CAD build for the part. Positions are in the model's coordinates, mm. A direction names the side the tool comes from. Coordinates: 2 decimals unless noted, no trailing zeros. Order: outer loops, then holes, each group sorted by start corner. A loop starts at its lowest first (then second) coordinate and runs counter-clockwise, first axis right, second up. Notation, with made-up numbers: M -12.75,63 L 32.25,63 A24 ccw 32.25,85 Z; hole C -21,-8.5 d2. An arc over 180 degrees is marked long. Write item = value, one per line. Start each with the question number.
```python
from build123d import *

# Parameters (mm, degrees)
SKETCH1_R               = 1.5875
BOSS_EXTRUDE1_DEPTH     = 22.86
TOP_CUT_DEPTH           = 8.255
BOTTOM_CUT_DEPTH        = 8.255
SKETCH5_R               = 10.033
CUT_EXTRUDE1_DEPTH      = 14.986
SKETCH7_R               = 2.032
CUT_EXTRUDE2_DEPTH      = 49.946539324
CUT_EXTRUDE3_REACH      = 50.947
CUT_EXTRUDE3_END_RADIUS = 10.033
SKETCH8_W               = 3.175
SKETCH8_H               = 6.35


with BuildPart() as part:
    # Sketch1 → Boss-Extrude1 (new body)
    with BuildSketch(Plane(origin=(0, 0, 0), x_dir=(1, 0, 0), z_dir=(0, 1, 0))):
        with BuildLine():
            Line((-6.35, -14.401477372), (-6.35, 2.54))
            Line((-6.35, 2.54), (-17.78, 2.54))
            Line((-17.78, 2.54), (-17.78, 25.4))
            Line((-17.78, 25.4), (0, 25.4))
            Line((0, 25.4), (0, -12.7))
            Line((0, -12.7), (12.7, -34.697045256))
            ThreePointArc((12.7, -34.697045256), (11.537869343, -39.034175913), (7.200738686, -37.872045256))
            Line((7.200738686, -37.872045256), (-6.35, -14.401477372))
        make_face()
        with Locations(Location((9.950369343, -36.284545256, 0), (0, 0, 270))):
            Circle(SKETCH1_R, mode=Mode.SUBTRACT)
        with Locations(Location((-2.749630657, -14.2875, 0), (0, 0, 270))):
            Circle(SKETCH1_R, mode=Mode.SUBTRACT)
    extrude(amount=BOSS_EXTRUDE1_DEPTH)

    # Sketch2 → Top Cut (cut)
    with BuildSketch(Plane(origin=(0, 22.86, 0), x_dir=(1, 0, 0), z_dir=(0, 1, 0))):
        Polygon((-6.35, -14.401477372), (8.788238686, -40.621675913), (14.2875, -37.446675913), (0, -12.7), (0, 2.54), (-6.35, 2.54), align=None)
    extrude(amount=-TOP_CUT_DEPTH, mode=Mode.SUBTRACT)

    # Sketch4 → Bottom Cut (cut)
    with BuildSketch(Plane.XZ):
        Polygon((-6.35, -2.54), (-6.35, 14.401477372), (8.788238686, 40.621675913), (14.2875, 37.446675913), (0, 12.7), (0, -2.54), align=None)
    extrude(amount=-BOTTOM_CUT_DEPTH, mode=Mode.SUBTRACT)

    # Sketch5 → Cut-Extrude1 (cut)
    with BuildSketch(Plane.ZY.offset(17.78)):
        with Locations((-13.97, 11.43)):
            Circle(SKETCH5_R)
    extrude(amount=-CUT_EXTRUDE1_DEPTH, mode=Mode.SUBTRACT)

    # Sketch7 → Cut-Extrude2 (cut, through all)
    with BuildSketch(Plane(origin=(0, 0, 0), x_dir=(0, 0, -1), z_dir=(1, 0, 0))):
        with Locations((13.97, 11.43)):
            Circle(SKETCH7_R)
    extrude(amount=-CUT_EXTRUDE2_DEPTH, mode=Mode.SUBTRACT)

    # Cut-Extrude3: up to this cylinder (the profile starts outside it)
    cut_extrude3_end = Plane(origin=(-4.7625, 11.43, -13.97), z_dir=(-1, 0, 0)) * Cylinder(CUT_EXTRUDE3_END_RADIUS, 122.96, mode=Mode.PRIVATE)
    # Sketch8 → Cut-Extrude3 (cut, up to the surface)
    with BuildSketch(Plane(origin=(0, 22.86, 0), x_dir=(1, 0, 0), z_dir=(0, 1, 0)), mode=Mode.PRIVATE) as cut_extrude3_sk1:
        with Locations((-4.7625, 13.97)):
            Rectangle(SKETCH8_W, SKETCH8_H)
    cut_extrude3_tool1 = extrude(cut_extrude3_sk1.sketch, amount=-CUT_EXTRUDE3_REACH, mode=Mode.PRIVATE) - cut_extrude3_end
    add(cut_extrude3_tool1.solids().sort_by_distance((-4.7625, 22.86, -13.97))[0], mode=Mode.SUBTRACT)


solid = part.part
```
1. Slice it at C-C (y = 10.25). Give the number of separate pieces and of enclosed holes in the cut face, plus the area to 3 significant figures.
2. 3-axis set-ups, long thin cutter, end or side, ignore diameter. For faces 1 (the flat face through (1, 8.255, 19)), 2 (the flat face through (-2.794, 9, -14)), 3 (the flat face through (-5, 22, -17.145)): which of +Z, -Z, +X, -X, +Y, -Y reach the whole face in a straight line?
3. Slice it at A-A (z = -13.97). Write the cut outline in (x, y) (3 decimals), plus the area to 3 significant figures.
4. Flat gauge pins, fed straight in: pin 1 (10 mm diameter, centred on x = -8.5, z = 19, fed in from +Y) (3 decimals); pin 2 (4 mm diameter, centred on x = 4.5, y = 12, fed in from -Z); pin 3 (6 mm diameter, centred on x = -4, z = 0.5, fed in from -Y) (3 decimals). Where does each tip first touch, or does it go through?
5. Probe L1, parallel to Z at x = -2, y = 19; L2, parallel to X at y = 12.5, z = -10.5; L3, parallel to Z at x = -5, y = 21 (3 decimals). List the from-to ranges inside material, lowest first.
6. Mould opens along X. For faces 4 (the flat face through (-5, 22, -10.795)), 5 (the flat face through (-9, 22.86, -14)), 6 (the flat face through (-6.35, 22, -14)), 7 (the flat face through (-6.35, 11, 6)) say: released by +X, released by -X, zero draft, split by the parting line, or undercut.
7. Slice it at D-D (x = -12). Write the cut outline in (y, z), plus the area to 3 significant figures.
8. Slice it at B-B (x = 9). Write the cut outline in (y, z) (3 decimals), plus the area to 3 significant figures.
Calculated:
q1.separate_pieces = 2
q1.enclosed_holes = 2
q1.area = 367 mm²
q2.face_1 = +Z, +X, -X, -Y
q2.face_2 = -X
q2.face_3 = +Y
q3.outline = M -17.78,0 L 0,0 L 0,9.398 L -2.794,9.398 L -2.794,1.397 L -17.78,1.397 Z; M -17.78,21.463 L -6.35,21.463 L -6.35,22.86 L -17.78,22.86 Z; M -3.175,21.463 L -2.794,21.463 L -2.794,13.462 L 0,13.462 L 0,22.86 L -3.175,22.86 Z
q3.area = 90.0 mm²
q4.pin_1 = 14.605
q4.pin_2 = 17.03
q4.pin_3 = 8.255
q5.L1 = -25.4 to -2.54
q5.L2 = -2.79 to 0
q5.L3 = -25.4 to -17.145, -10.795 to -2.54
q6.face_4 = undercut
q6.face_5 = zero draft
q6.face_6 = undercut
q6.face_7 = released by -X
q7.outline = M 0,-25.4 L 22.86,-25.4 L 22.86,-2.54 L 0,-2.54 Z; hole C 11.43,-13.97 d20.07
q7.area = 206 mm²
q8.outline = M 8.255,28.288 L 14.605,28.288 L 14.605,35.013 L 8.255,35.013 Z; M 8.255,37.556 L 14.605,37.556 L 14.605,39.314 L 8.255,39.314 Z
q8.area = 53.9 mm²
